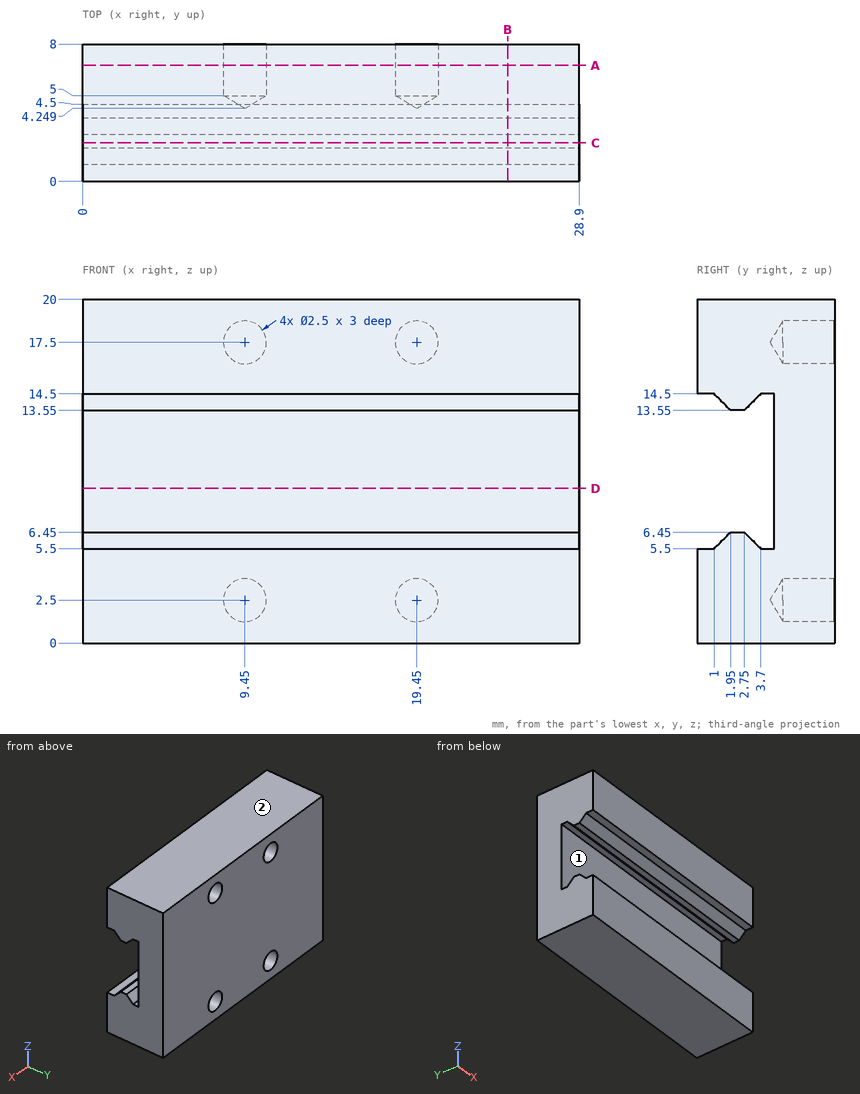
Can you work these out from the drawing? Everything is in mm from the part's minimum corner. A direction names the side the tool comes from. Coordinates: 2 decimals unless noted, no trailing zeros. Write each loop counter-clockwise with the first axis right and the second up, starting at its lowest first coordinate (ties: lowest second). Pieces come first, ordered by that corner, then holes. Notation, with made-up numbers: (83, 24) -> (117, 24) arc R14 ccw to (117, 33) -> close; hole circle Ø8 at (89.5, 52). An arc over 180 degrees is marked (long way). Write each question's results on one line, items separated by ' | '. Start each with the question number.
Item 1: If we section it at C-C, the plane y = 2.25: Write out the boundary of the cut face in (x, z), and give its area (3 significant figures).
Item 2: Please list where these lines run through material, in increasing order: probe 1 along X at (y, z) = (6.5, 17.5); probe 2 along Z at (x, y) = (9.45, 7.15); probe 3 along Z at (x, y) = (9, 0.5).
Item 3: If we section it at B-B, the plane x = 24.75: Write out the boundary of the cut face in (y, z).
Item 4: If we section it at A-A, the plane y = 6.75: Write out the boundary of the cut face in (x, z).
Item 5: I'm going to push flat-ended pins straight in: P1, Ø7, axis at x = 11, z = 10, coming from the -Y side; P2, Ø2, axis at x = 19.45, z = 2.5, coming from the +Y side. Where does each tip first touch, or does it pass through?
Item 6: On a 3-axis mill with a long thin cutter (end or side, diameter ignored), from which of +Z, -Z, +X, -X, +Y, -Y can I reach the whole of each face in a straight line? I mean the marked faces 1 and 2. Say none if no direction works.
Item 7: If we section it at D-D, the plane z = 9: Write out the boundary of the cut face in (x, y), and give its area (3 significant figures).
Answer block:
1) outline: (0, 0) -> (28.9, 0) -> (28.9, 6.45) -> (0, 6.45) -> close; (0, 13.55) -> (28.9, 13.55) -> (28.9, 20) -> (0, 20) -> close | area: 373 mm²
2) probe 1: 0 to 8.2, 10.7 to 18.2, 20.7 to 28.9 | probe 2: 0 to 1.25, 3.75 to 16.25, 18.75 to 20 | probe 3: 0 to 5.5, 14.5 to 20
3) outline: (0, 0) -> (8, 0) -> (8, 20) -> (0, 20) -> (0, 14.5) -> (1, 14.5) -> (1.95, 13.55) -> (2.75, 13.55) -> (3.7, 14.5) -> (4.5, 14.5) -> (4.5, 5.5) -> (3.7, 5.5) -> (2.75, 6.45) -> (1.95, 6.45) -> (1, 5.5) -> (0, 5.5) -> close
4) outline: (0, 0) -> (28.9, 0) -> (28.9, 20) -> (0, 20) -> close; hole circle Ø2.5 at (9.45, 2.5); hole circle Ø2.5 at (9.45, 17.5); hole circle Ø2.5 at (19.45, 2.5); hole circle Ø2.5 at (19.45, 17.5)
5) P1: y = 4.5 | P2: y = 4.85
6) face 1: +X, -X | face 2: +Z, +X, -X, +Y, -Y
7) outline: (0, 4.5) -> (28.9, 4.5) -> (28.9, 8) -> (0, 8) -> close | area: 101 mm²
